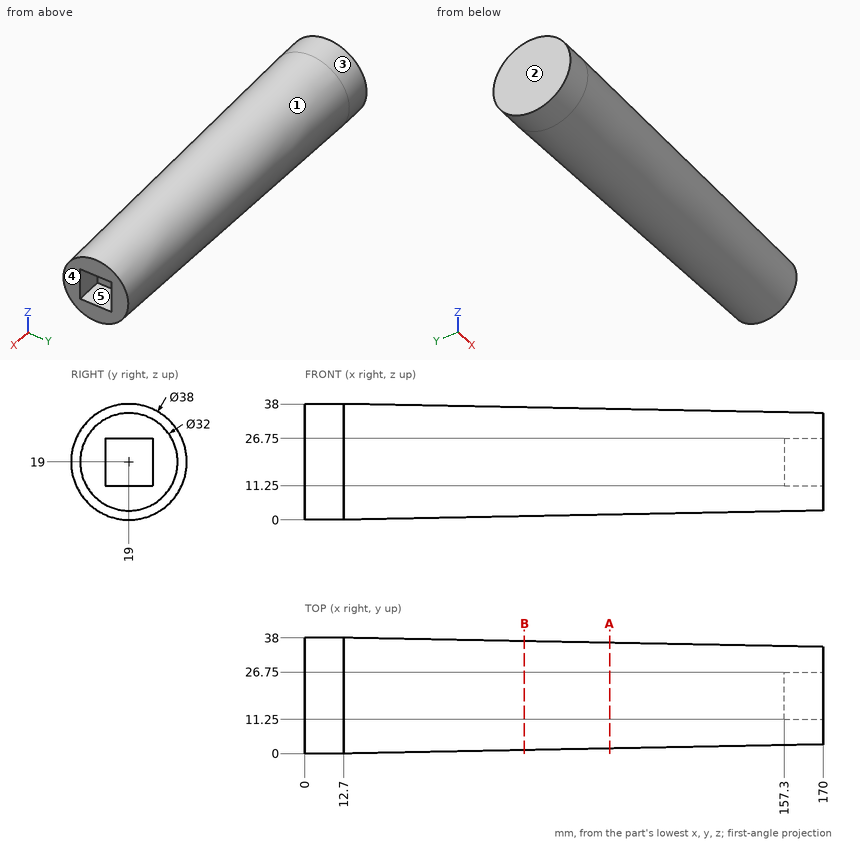
Print and shaded views of the part. All mm, measured from the part's lowest x, y and z. A direction names the side the tool comes from. Coordinates: 2 decimals unless noted, no trailing zeros. Order: outer loops, then holes, each group sorted by start corner. A loop starts at its lowest first (then second) coordinate and runs counter-clockwise, first axis right, second up. Notation, with made-up numbers: (84, 30.25) -> (141, 30.25) arc R31 ccw to (141, 58.25) -> close; hole circle Ø2 at (-39.5, 83). An arc over 180 degrees is marked (long way). Answer as a JSON object with one key per item and string values. Group by question number.
1) Pull direction Z, two halves, no side cores. Call the marked faces 3, 4 and 5: +Z half, -Z half, draft (parallel to the pull), parting line (faces both ways), or undercut.
2) Flat gauge pins, fed straight in: pin 1 (8 mm diameter, centred on x = 111, y = 23.5, fed in from +Z); pin 2 (3 mm diameter, centred on y = 29, z = 24, fed in from -X); pin 3 (4.5 mm diameter, centred on y = 16.5, z = 19, fed in from +X); pin 4 (1 mm diameter, centred on x = 145, y = 16.5, fed in from -Z). Where does each tip first touch, or does it go through?
3) Cut at B-B, the plane x = 72. Write the cut outline in (y, z), then the cut area to 3 significant figures.
4) Drill centre lines: L1, parallel to Z at x = 27.5, y = 6; L2, parallel to Z at x = 58, y = 26.5; L3, parallel to Y at x = 72.5, z = 3. Where is each one in solid material? Low to high.
5) Cut at A-A, the plane x = 100. Write the cut outline in (y, z), then the cut area to 3 significant figures.
6) Which spindle directions (+Z, -Z, +X, -X, +Y, -Y) get a long thin tool onto all of the face, cutting with end or side? Do the marked faces 1 and 2. Say none if no direction does.
Check values:
{
 "1": {"face 3": "parting line", "face 4": "draft", "face 5": "undercut"},
 "2": {"pin 1": "stops at z = 36.14", "pin 2": "stops at x = 0", "pin 3": "stops at x = 157.3", "pin 4": "stops at z = 2.64"},
 "3": {"outline": "circle Ø35.74 at (19, 19)", "area": "1,000 mm²"},
 "4": {"L1": "z = 5.53 to 32.47", "L2": "z = 2.49 to 35.51", "L3": "y = 11.07 to 26.93"},
 "5": {"outline": "circle Ø34.67 at (19, 19)", "area": "944 mm²"},
 "6": {"face 1": "+X", "face 2": "+Z, -Z, -X, +Y, -Y"}
}
